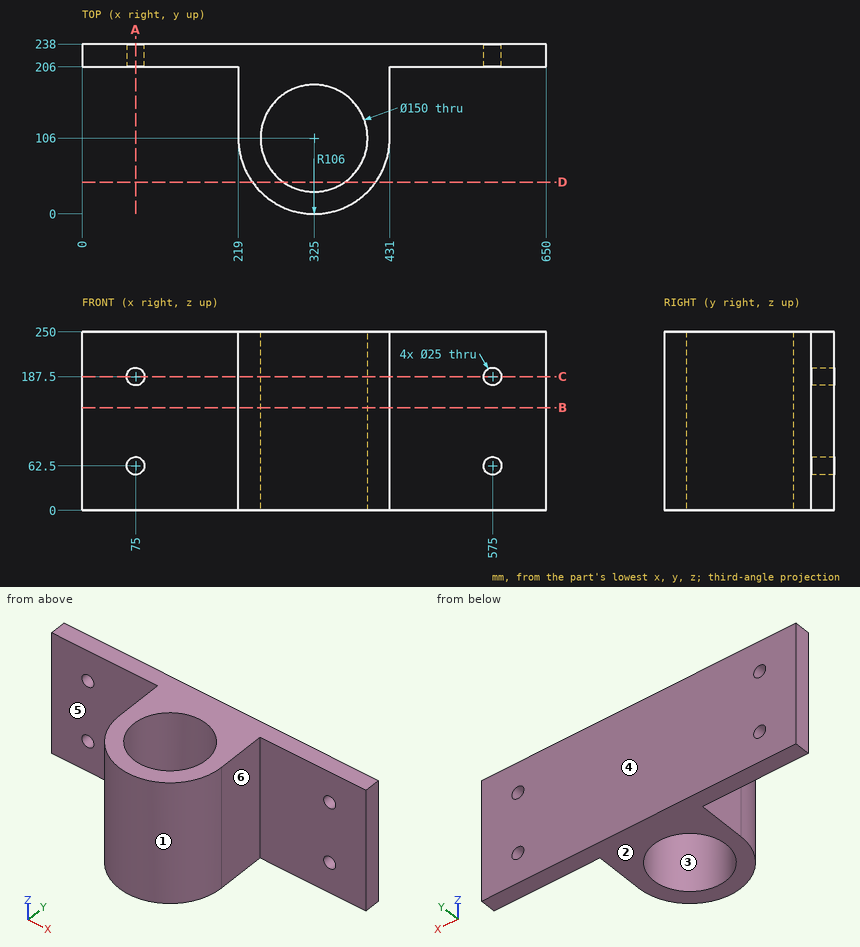
Geometry: see drawing. Coordinates: mm, zero at the bounding-box minimum. A direction names the side the tool comes from. Round coordinates to 2 decimals unless told otherwise and drop trailing zeros. Order: outer loops, then holes, each group sorted by start corner. A loop starts at its lowest first (then second) coordinate and runs counter-clockwise, first axis right, second up. Notation, with made-up numbers: (59, 66) - (102, 66) arc R16 cw to (102, 93) - close; hole circle Ø2 at (29.5, 48.25). An arc over 180 degrees is marked (long way). One line per question, with ' | ' between items. Start each with the question number.
1) Ray query, probe 1 along Z at (x, y) = (75, 221); probe 2 along X at (y, z) = (218, 187); probe 3 along Y at (x, z) = (325, 95). Return the intervals inside material, ascending.
2) Cut plane B-B, the plane z = 144. Return the cut outline in (x, y).
3) Cut plane A-A, the plane x = 75. Return the cut outline in (y, z), then the cut area to 3 significant figures.
4) Cut plane C-C, the plane z = 187.5. Return the cut outline in (x, y), then the cut area to 3 significant figures.
5) Pull-direction query (Y, two-part tool) for the marked faces 1, 2 and 3; classes: +Y half, -Y half, draft (parallel to the pull), parting line (faces both ways), or undercut.
6) Set-up query: the marked faces 4, 5 and 6. Return all of +Z, -Z, +X, -X, +Y, -Y with unobstructed straight access to the full face (end or side cutting, diameter ignored); none if empty.
7) Contact query for flat-ended pins moving along their axis: P1, Ø1, axis at y = 67.5, z = 222.5, coming from the +X side; P2, Ø3, axis at y = 47.5, z = 156.5, coming from the -X side; P3, Ø8, axis at y = 78.5, z = 169, coming from the +X side; P4, Ø20, axis at x = 575, z = 187.5, coming from the +Y side. Output: stop coordinate, or through.
8) Cut plane D-D, the plane y = 44.5. Return the cut outline in (x, z), then the cut area to 3 significant figures.
Worked out:
1) probe 1: z = 0 to 50, 75 to 175, 200 to 250 | probe 2: x = 0 to 62.51, 87.49 to 562.51, 587.49 to 650 | probe 3: y = 0 to 31, 181 to 238
2) outline: (0, 206) - (219, 206) - (219, 106) arc R106 ccw to (431, 106) - (431, 206) - (650, 206) - (650, 238) - (0, 238) - close; hole circle Ø150 at (325, 106)
3) outline: (206, 0) - (238, 0) - (238, 50) - (206, 50) - close; (206, 75) - (238, 75) - (238, 175) - (206, 175) - close; (206, 200) - (238, 200) - (238, 250) - (206, 250) - close | area: 6,400 mm^2
4) outline: (0, 206) - (62.5, 206) - (62.5, 238) - (0, 238) - close; (87.5, 206) - (219, 206) - (219, 106) arc R106 ccw to (431, 106) - (431, 206) - (562.5, 206) - (562.5, 238) - (87.5, 238) - close; (587.5, 206) - (650, 206) - (650, 238) - (587.5, 238) - close; hole circle Ø150 at (325, 106) | area: 40,400 mm^2
5) face 1: -Y half | face 2: draft | face 3: undercut
6) face 4: +Z, -Z, +X, -X, +Y | face 5: +Z, -Z, -X, -Y | face 6: +Z, -Z, +X, -Y
7) P1: stops at x = 423.95 | P2: stops at x = 235.63 | P3: stops at x = 428.36 | P4: passes through
8) outline: (238.66, 0) - (282.07, 0) - (282.07, 250) - (238.66, 250) - close; (367.93, 0) - (411.34, 0) - (411.34, 250) - (367.93, 250) - close | area: 21,700 mm^2
